```python
from build123d import *

# Parameters (mm, degrees)
SKETCH1_W           = 1000
SKETCH1_H           = 1000
BOSS_EXTRUDE1_DEPTH = 40
SKETCH2_W           = 1000
SKETCH2_H           = 600
CUT_EXTRUDE1_DEPTH  = 20
SKETCH6_R           = 25
BOSS_EXTRUDE8_DEPTH = 800
SKETCH7_W           = 30
SKETCH7_H           = 30
CUT_EXTRUDE3_DEPTH  = 50
SKETCH8_R           = 8
CUT_EXTRUDE4_DEPTH  = 30
CUT_EXTRUDE5_START  = -30
SKETCH9_R           = 8
CUT_EXTRUDE5_DEPTH  = 30
SKETCH10_W          = 50
SKETCH10_H          = 600
CUT_EXTRUDE6_DEPTH  = 30
CUT_EXTRUDE7_DEPTH  = 30


with BuildPart() as part:
    # Sketch1 → Boss-Extrude1 (new body)
    with BuildSketch(Plane(origin=(0, 0, 0), x_dir=(1, 0, 0), z_dir=(0, 1, 0))):
        with Locations((500, -500)):
            Rectangle(SKETCH1_W, SKETCH1_H)
    extrude(amount=BOSS_EXTRUDE1_DEPTH)

    # Sketch2 → Cut-Extrude1 (cut)
    with BuildSketch(Plane(origin=(0, 40, 0), x_dir=(1, 0, 0), z_dir=(0, 1, 0))):
        with Locations((500, -500)):
            Rectangle(SKETCH2_W, SKETCH2_H)
    extrude(amount=-CUT_EXTRUDE1_DEPTH, mode=Mode.SUBTRACT)

    # Sketch6 → Boss-Extrude8 (add)
    with BuildSketch(Plane(origin=(0, 0, 0), x_dir=(-1, 0, 0), z_dir=(0, -1, 0))):
        with Locations(Location((-50, -950, 0), (0, 0, 90))):
            Circle(SKETCH6_R)
        with Locations(Location((-950, -950, 0), (0, 0, 90))):
            Circle(SKETCH6_R)
        with Locations(Location((-950, -50, 0), (0, 0, 90))):
            Circle(SKETCH6_R)
        with Locations(Location((-50, -50, 0), (0, 0, 90))):
            Circle(SKETCH6_R)
    extrude(amount=BOSS_EXTRUDE8_DEPTH)

    # Sketch7 → Cut-Extrude3 (cut)
    with BuildSketch(Plane(origin=(0, 40, 0), x_dir=(1, 0, 0), z_dir=(0, 1, 0))):
        with Locations((25, -175)):
            Rectangle(SKETCH7_W, SKETCH7_H)
        with Locations((25, -825)):
            Rectangle(SKETCH7_W, SKETCH7_H)
    extrude(amount=-CUT_EXTRUDE3_DEPTH, mode=Mode.SUBTRACT)

    # Sketch8 → Cut-Extrude4 (cut)
    with BuildSketch(Plane.XY.offset(200)):
        with Locations((25, 30)):
            Circle(SKETCH8_R)
    extrude(amount=-CUT_EXTRUDE4_DEPTH, mode=Mode.SUBTRACT)

    # Sketch9 → Cut-Extrude5 (cut)
    with BuildSketch(Plane(origin=(0, 0, 800), x_dir=(-1, 0, 0), z_dir=(0, 0, -1)).offset(CUT_EXTRUDE5_START)):
        with Locations(Location((-25, 30, 0), (0, 0, 180))):
            Circle(SKETCH9_R)
    extrude(amount=CUT_EXTRUDE5_DEPTH, mode=Mode.SUBTRACT)

    # Sketch10 → Cut-Extrude6 (cut)
    with BuildSketch(Plane(origin=(0, 20, 0), x_dir=(1, 0, 0), z_dir=(0, 1, 0))):
        with Locations((25, -500)):
            Rectangle(SKETCH10_W, SKETCH10_H)
    extrude(amount=-CUT_EXTRUDE6_DEPTH, mode=Mode.SUBTRACT)

    # Sketch11 → Cut-Extrude7 (cut)
    with BuildSketch(Plane(origin=(0, 40, 0), x_dir=(1, 0, 0), z_dir=(0, 1, 0))):
        Polygon((700, -115), (900, -115), (900, -100), (900, -85), (700, -85), align=None)
    extrude(amount=-CUT_EXTRUDE7_DEPTH, mode=Mode.SUBTRACT)


solid = part.part
```
Could you check a few things on this model? Use its own coordinates, in mm. A direction names the side the tool comes from. Coordinates: 2 decimals unless noted, no trailing zeros. Loops run counter-clockwise (first coordinate to the right, second up) from the corner with the lowest first, then second, coordinate; pieces in that order, holes last. Notation, with made-up numbers: M 19.25,6 L 50.25,6 A23 ccw 50.25,39 Z; hole C 15.25,58 d1. An arc over 180 degrees is marked long. Put each result on its own line as item: value. Start each with the question number.
(1) Thinking about a two-plate mould opening in Z: for faces 4 (the face through (25, 20, 160)), 5 (the face through (50, -800, 50)), 6 (the face through (518, 20, 496)), 7 (the face through (493, 20, 0)), which applies, pulls with the +Z half, pulls with the -Z half, needs draft (parallel to the pull), parting line crosses it, or undercut?
(2) Will these pins go through, and if not, where does the flat tip stop? P1, Ø16, axis at y = 11, z = 609.5, coming from the -X side; P2, Ø3, axis at x = 291.5, z = 249.5, coming from the -Y side.
(3) For faces 1 (the face through (25.594, -394.4, 55.42)), 2 (the face through (799, 25, 115)), 3 (the face through (25, 20, 840)), which set-ups out of +Z, -Z, +X, -X, +Y, -Y let a thin tool reach every point of the face, with its end or its side?
(4) Suppose I cut it at B-B on y = -628. Please give me the cut outline in (x, z), then the cut area to 3 significant figures.
(5) Suppose I cut it at C-C on z = 950. Please give me the cut outline in (x, y), then the cut area to 3 significant figures.
(6) I need wall thicknesses on line 1 (Y direction, x = 25, z = 198); line 2 (X direction, y = 30, z = 803); line 3 (Y direction, x = 859.5, z = 938). Which ranges of each line are inside material? Lowest first, please. Write a range as from..to.
(7) Suppose I cut it at D-D on x = 950. Please give me the cut outline in (y, z).
(8) Suppose I cut it at A-A on x = 129. Please give me the cut outline in (y, z), then the cut area to 3 significant figures.
Solutions:
1. face 4: undercut
1. face 5: needs draft
1. face 6: undercut
1. face 7: pulls with the -Z half
2. P1: stops at x = 50
2. P2: stops at y = 0
3. face 1: -Y
3. face 2: +Y
3. face 3: +Y, -Y
4. outline: C 50,50 d50; C 50,950 d50; C 950,50 d50; C 950,950 d50
4. area: 7,850 mm2
5. outline: M 0,0 L 25,0 L 25,-800 L 75,-800 L 75,0 L 925,0 L 925,-800 L 975,-800 L 975,0 L 1000,0 L 1000,40 L 0,40 Z
5. area: 120,000 mm2
6. line 1: y = 0..22, 38..40
6. line 2: x = 0..17, 33..1000
6. line 3: y = 0..40
7. outline: M -800,25 L 0,25 L 0,0 L 40,0 L 40,200 L 20,200 L 20,800 L 40,800 L 40,1000 L 0,1000 L 0,975 L -800,975 L -800,925 L 0,925 L 0,75 L -800,75 Z
8. outline: M 0,0 L 40,0 L 40,200 L 20,200 L 20,800 L 40,800 L 40,1000 L 0,1000 Z
8. area: 28,000 mm2
